Can you work these out from the model? Positions are in its coordinate system, mm. A direction names the side the tool comes from. Coordinates: 2 decimals unless noted, no trailing zeros. Order: outer loops, then holes, each group sorted by start corner. A loop starts at its lowest first (then second) coordinate and runs counter-clockwise, first axis right, second up. Notation, with made-up numbers: (50.25, 56) -> (92.25, 56) arc R16 ccw to (92.25, 65) -> close; hole circle Ø10 at (89.25, 52.5). An arc over 180 degrees is marked (long way). Write item = value, one per line.
Autodesk Inventor part; units mm, degrees
ref_plane "YZ Plane" through (0, 0, 0) normal (1, 0, 0) x (0, 1, 0)
ref_plane "XZ Plane" through (0, 0, 0) normal (0, 1, 0) x (-1, 0, 0)
ref_plane "XY Plane" through (0, 0, 0) normal (0, 0, 1) x (1, 0, 0)
sketch "Sketch1" plane through (0, 0, 0) normal (0, 1, 0) x (-1, 0, 0)
  circle A0 centre (0, 0) radius 4
  dimension "d0" = 8
extrude "Extrusion1" add sketch "Sketch1" along normal blind 5.08
sketch "Sketch2" plane through (0, 5.08, 0) normal (0, 1, 0) x (1, 0, 0)
  circle A0 centre (0, 0) radius 6.35
  dimension "d3" = 12.7
extrude "Extrusion2" add sketch "Sketch2" along normal blind 5.08
sketch "Sketch3" plane through (0, 10.16, 0) normal (0, 1, 0) x (1, 0, 0)
  circle A0 centre (0, 0) radius 2.3813
  circle A1 centre (0, 0) radius 2.3813
  point P0 (0, 0)
extrude "Extrusion3" cut sketch "Sketch3" against normal through all
properties part number "Shaft_Adapter"
Item 1: I'm going to push flat-ended pins straight in: P1, Ø4, axis at x = 0, z = 0, coming from the +Y side; P2, Ø5, axis at x = -3, z = 2, coming from the -Y side; P3, Ø3, axis at y = 1, z = 0.5, coming from the +X side; P4, Ø2, axis at y = 1.5, z = -3.5, coming from the +X side. Where does each tip first touch, or does it pass through?
A:
P1 = through
P2 = 0
P3 = 4
P4 = 3.12
Item 2: If we mould it in two halves opening along X, with no side actions, what happens to faces 1 (the cylindrical face through (0.867, 2.504, 3.905)), 2 (the flat face through (-2, 0, -2)), 3 (the cylindrical face through (1.1, 5.15, 2.11))? For each: pulls with the +X half, pulls with the -X half, needs draft (parallel to the pull), parting line crosses it, or undercut.
A:
face_1 = parting line crosses it
face_2 = needs draft
face_3 = undercut
Item 3: I want a section at A-A, the plane x = 0. Please give me the cut outline in (y, z), plus the area to 3 significant figures.
A:
outline = (0, -4) -> (5.08, -4) -> (5.08, -6.35) -> (10.16, -6.35) -> (10.16, -2.38) -> (0, -2.38) -> close; (0, 2.38) -> (10.16, 2.38) -> (10.16, 6.35) -> (5.08, 6.35) -> (5.08, 4) -> (0, 4) -> close
area = 56.8 mm2
Item 4: I want a section at D-D, the plane x = 3.75. Please give me the cut outline in (y, z).
A:
outline = (0, -1.39) -> (5.08, -1.39) -> (5.08, -5.12) -> (10.16, -5.12) -> (10.16, 5.12) -> (5.08, 5.12) -> (5.08, 1.39) -> (0, 1.39) -> close
Item 5: I want a section at B-B, the plane z = 0. Please give me the cut outline in (x, y), plus the area to 3 significant figures.
A:
outline = (-6.35, 5.08) -> (-4, 5.08) -> (-4, 0) -> (-2.38, 0) -> (-2.38, 10.16) -> (-6.35, 10.16) -> close; (2.38, 0) -> (4, 0) -> (4, 5.08) -> (6.35, 5.08) -> (6.35, 10.16) -> (2.38, 10.16) -> close
area = 56.8 mm2
Item 6: If I drill on probe 1 along X at (y, z) = (5.25, 0); probe 2 along Z at (x, y) = (0, 2.5), over which ranges is the centre line in solid material (lowest first)?
A:
probe_1 = -6.35 to -2.38, 2.38 to 6.35
probe_2 = -4 to -2.38, 2.38 to 4
Item 7: I want a section at C-C, the plane y = 5.75. Please give me the cut outline in (x, z), plus the area to 3 significant figures.
A:
outline = circle Ø12.7 at (0, 0); hole circle Ø4.76 at (0, 0)
area = 109 mm2
Item 8: For faces 4 (the flat face through (1.3, 5.08, 4.1)), 5 (the cylindrical face through (-1.38, 7.58, -6.2)), which set-ups out of +Z, -Z, +X, -X, +Y, -Y let a thin tool reach every point of the face, with its end or its side?
A:
face_4 = -Y
face_5 = +Y, -Y
